```python
from build123d import *

# Parameters (mm, degrees)
F1_DEPTH = 12.5
F2_R     = 4.907825
F3_DEPTH = 40.001
F4_W     = 8.482946
F4_H     = 9.896773
F5_DEPTH = 25


with BuildPart() as f1:
    # F0 (on Front) → F1 (new body, symmetric)
    with BuildSketch(Plane.XZ):
        Polygon((-26.978808, 25.542999), (-26.978808, 7.346645), (33.021192, 7.346645), (33.021192, 24.45209), (13.021192, 24.45209), (13.021192, 44.452089), (-6.978808, 44.452089), (-6.978808, 25.542999), align=None)
    extrude(amount=F1_DEPTH, both=True)

    # F2 (on face) → F3 (cut, through all)
    with BuildSketch(Plane.YZ.offset(13.021192)):
        with Locations((0, 31.952426)):
            Circle(F2_R)
    extrude(amount=-F3_DEPTH, mode=Mode.SUBTRACT)

    # F4 (on face) → F5 (join)
    with BuildSketch(Plane.XY.offset(24.45209)):
        with Locations((23.586721, 0)):
            Rectangle(F4_W, F4_H)
    extrude(amount=F5_DEPTH)


solid = f1.part
```
Check sheet for the modelled part. Datum: model origin and axes. Units: mm. A direction names the side the tool comes from. Coordinates: 2 decimals unless noted, no trailing zeros. Order: outer loops, then holes, each group sorted by start corner. A loop starts at its lowest first (then second) coordinate and runs counter-clockwise, first axis right, second up. Notation, with made-up numbers: M 45,-16.5 L 52,-16.5 A20 ccw 52,13.5 Z; hole C 18.25,59.5 d10. An arc over 180 degrees is marked long. Write each question's results on one line, items separated by ' | '. Start each with the question number.
1. Cross-section at A-A on y = 0. Record the cut outline in (x, z).
2. Mould release check, pull along X, two halves, no side actions. Record for faces 1 (the face through (13.021, -3, 37)), 2 (the face through (3.16, -1.06, 27.16)), 3 (the face through (19, 0, 24.452)), 4 (the face through (-6.979, -0.2, 37.2)): +X half, -X half, draft (parallel to the pull), parting line (faces both ways), or undercut.
3. Cross-section at C-C on x = 24.5. Record the cut outline in (y, z), and give its area (3 significant figures).
4. Go/stop test with flat-tipped pins: P1, Ø2.5, axis at x = 22.5, z = 36, coming from the +Y side; P2, Ø15, axis at y = 5, z = 38, coming from the -X side; P3, Ø7, axis at x = 25, z = 35.5, coming from the -Y side. Record where each tip stops, or that it passes through.
5. Cross-section at D-D on z = 46. Record the cut outline in (x, y).
6. Access from +Z, -Z, +X, -X, +Y, -Y to the whole of each face (thin tool, end or side, straight path). Record for faces 5 (the face through (24, -4.948, 37)), 6 (the face through (19.345, 0, 37)), 7 (the face through (27.828, 0, 37)).
7. Cross-section at B-B on y = 9.25. Record the cut outline in (x, z).
8. Material ranges on probe 1 along Z at (x, y) = (0.25, 0); probe 2 along X at (y, z) = (-1, 24.5); probe 3 along Z at (x, y) = (-1, 5.5), recorded low to high.
Checks:
1) outline: M -26.98,7.35 L 33.02,7.35 L 33.02,24.45 L 27.83,24.45 L 27.83,49.45 L 19.35,49.45 L 19.35,24.45 L 13.02,24.45 L 13.02,27.04 L -6.98,27.04 L -6.98,25.54 L -26.98,25.54 Z; M -6.98,36.86 L 13.02,36.86 L 13.02,44.45 L -6.98,44.45 Z
2) face 1: undercut | face 2: draft | face 3: undercut | face 4: -X half
3) outline: M -12.5,7.35 L 12.5,7.35 L 12.5,24.45 L 4.95,24.45 L 4.95,49.45 L -4.95,49.45 L -4.95,24.45 L -12.5,24.45 Z | area: 675 mm²
4) P1: stops at y = 4.95 | P2: stops at x = -6.98 | P3: stops at y = -4.95
5) outline: M 19.35,-4.95 L 27.83,-4.95 L 27.83,4.95 L 19.35,4.95 Z
6) face 5: +Z, +X, -Y | face 6: +Z, +Y, -Y | face 7: +Z, +X, +Y, -Y
7) outline: M -26.98,7.35 L 33.02,7.35 L 33.02,24.45 L 13.02,24.45 L 13.02,44.45 L -6.98,44.45 L -6.98,25.54 L -26.98,25.54 Z
8) probe 1: z = 7.35 to 27.04, 36.86 to 44.45 | probe 2: x = -26.98 to 13.02, 19.35 to 27.83 | probe 3: z = 7.35 to 44.45
